```python
from build123d import *

# Parameters (mm, degrees)
SKETCH1_R                        = 5
BOSS_EXTRUDE1_DEPTH              = 34
CHAMFER1_SIZE                    = 0.5
SKETCH2_R                        = 11
BOSS_EXTRUDE2_DEPTH              = 2
SKETCH3_W                        = 3
SKETCH3_H                        = 1.8
CUT_EXTRUDE1_DEPTH               = 12
FILLET1_R                        = 1.5
BOSS_EXTRUDE3_START              = 10
SKETCH4_R                        = 5
BOSS_EXTRUDE3_DEPTH              = 10
SKETCH6_W                        = 0.8
SKETCH6_H                        = 0.5
CHAMFER2_SIZE                    = 0.5
CUT_EXTRUDE2_DEPTH               = 38.389838192
TAP_DRILL_FOR_M4_HELICOIL1_D     = 4.2
TAP_DRILL_FOR_M4_HELICOIL1_DEPTH = 20
TAP_DRILL_FOR_M4_HELICOIL1_TIP   = 1.2618073


with BuildPart() as part:
    # Sketch1 → Boss-Extrude1 (new body)
    with BuildSketch(Plane(origin=(0, 0, 0), x_dir=(0, 0, -1), z_dir=(1, 0, 0))):
        Circle(SKETCH1_R)
    extrude(amount=BOSS_EXTRUDE1_DEPTH)

    # Chamfer1
    chamfer1_edges = [part.edges().sort_by_distance(p)[0] for p in [
        (34, 0, 5),
    ]]
    chamfer(chamfer1_edges, length=CHAMFER1_SIZE)

    # Sketch2 → Boss-Extrude2 (add)
    with BuildSketch(Plane.ZY):
        Circle(SKETCH2_R)
    extrude(amount=BOSS_EXTRUDE2_DEPTH)

    # Sketch3 → Cut-Extrude1 (cut)
    with BuildSketch(Plane(origin=(34, 0, 0), x_dir=(0, 0, -1), z_dir=(1, 0, 0))):
        with Locations((0, 4.1)):
            Rectangle(SKETCH3_W, SKETCH3_H)
    extrude(amount=-CUT_EXTRUDE1_DEPTH, mode=Mode.SUBTRACT)

    # Fillet1
    fillet1_edges = [part.edges().sort_by_distance(p)[0] for p in [
        (22, 3.984848004, 1.5),
        (22, 3.984848004, -1.5),
    ]]
    fillet(fillet1_edges, radius=FILLET1_R - 0.0001)  # a hair under: the kernel refuses the full size

    # Sketch4 → Boss-Extrude3 (add)
    with BuildSketch(Plane.ZY.offset(2).offset(BOSS_EXTRUDE3_START)):
        with Locations(Location((0, 0, 0), (0, 0, 72.542396876))):
            Circle(SKETCH4_R)
    extrude(amount=-BOSS_EXTRUDE3_DEPTH)

    # Sketch6 → Cut-Revolve1 (revolve, cut)
    with BuildSketch(Plane.XY, mode=Mode.PRIVATE) as cut_revolve1_sk:
        with Locations((-2.4, 4.75)):
            Rectangle(SKETCH6_W, SKETCH6_H)
        with Locations((0.4, 4.75)):
            Rectangle(SKETCH6_W, SKETCH6_H)
    revolve(cut_revolve1_sk.sketch.rotate(Axis((0, 0, 0), (1, 0, 0)), 90), axis=Axis((0, 0, 0), (1, 0, 0)), mode=Mode.SUBTRACT)

    # Chamfer2
    chamfer2_edges = [part.edges().sort_by_distance(p)[0] for p in [
        (-12, -4.769696007, -1.5),
    ]]
    chamfer(chamfer2_edges, length=CHAMFER2_SIZE)

    # Sketch7 → Cut-Extrude2 (cut, through all)
    with BuildSketch(Plane(origin=(0, 0, 0), x_dir=(0, 0, -1), z_dir=(1, 0, 0))):
        with BuildLine():
            Line((-4, 3), (-4, -3))
            ThreePointArc((-4, -3), (-5, 0), (-4, 3))
        make_face()
        with BuildLine():
            Line((4, 3), (4, -3))
            ThreePointArc((4, -3), (5, 0), (4, 3))
        make_face()
    extrude(amount=CUT_EXTRUDE2_DEPTH, mode=Mode.SUBTRACT)

    # Tap Drill for M4 Helicoil1
    with Locations(Plane(origin=(34, 0, 0), x_dir=(0, 0, -1), z_dir=(1, 0, 0))):
        with Locations((0, 0)):
            Hole(TAP_DRILL_FOR_M4_HELICOIL1_D / 2, depth=TAP_DRILL_FOR_M4_HELICOIL1_DEPTH)
            with Locations((0, 0, -(TAP_DRILL_FOR_M4_HELICOIL1_DEPTH + TAP_DRILL_FOR_M4_HELICOIL1_TIP / 2))):  # 118° drill point
                Cone(0, TAP_DRILL_FOR_M4_HELICOIL1_D / 2, TAP_DRILL_FOR_M4_HELICOIL1_TIP, mode=Mode.SUBTRACT)


solid = part.part
```
Geometry check sheet. Reference: the model listing, model coordinates, mm. A direction names the side the tool comes from. Give positions to 0.01 mm unless a question says otherwise; leave off trailing zeros. Loops run counter-clockwise (first coordinate to the right, second up) from the corner with the lowest first, then second, coordinate; pieces in that order, holes last. Notation, with made-up numbers: (34, 19.5) - (46, 19.5) arc R21 ccw to (46, 42.5) - close; hole circle Ø7 at (64, -5). An arc over 180 degrees is marked (long way). Use CSV: the item, a comma, the result in double quotes. Start each with the question number.
Q1. Section check C-C, the plane x = 4. Record the cut outline in (y, z), and give its area (3 significant figures).
Q2. Section check B-B, the plane y = 5.5. Record the cut outline in (x, z), and give its area (3 significant figures).
Q3. Section check A-A, the plane x = 25. Record the cut outline in (y, z), and give its area (3 significant figures).
Q4. Scan lines: probe 1 along Z at (x, y) = (19.75, 0); probe 2 along Z at (x, y) = (24, 4); probe 3 along X at (y, z) = (8, 5.75). Record each from-to range of solid material in increasing order. Write a range as from..to.
Q5. Access from +Z, -Z, +X, -X, +Y, -Y to the whole of each face (thin tool, end or side, straight path). Record for faces 4 (the face through (-2.39, -3.04, -3.32)), 5 (the face through (0.4, -4.5, 0.1)), 6 (the face through (0.4, 4.5, -0.1)), 7 (the face through (23.86, 0.631, 2.003)).
Q6. Go/stop test with flat-tipped pins: pin 1 Ø2 at (x, y) = (1.5, 3) entering from -Z; pin 2 Ø5 at (x, y) = (26, -0.5) entering from +Z; pin 3 Ø2 at (x, z) = (24, 0.5) entering from -Y. Record where each tip stops, or that it passes through.
Q7. Release check for a two-part mould opening along X. For faces 1 (the face through (-12, 0, 0)), 2 (the face through (0.8, 4.7, 0)), 3 (the face through (29, 4, -1.5)) record: +X half, -X half, draft (parallel to the pull), parting line (faces both ways), or undercut.
Findings below:
1,outline,"(-3, -4) - (3, -4) arc R5 ccw to (3, 4) - (-3, 4) arc R5 ccw to start"
1,area,"70.4 mm^2"
2,outline,"(-2, -9.53) - (0, -9.53) - (0, 9.53) - (-2, 9.53) - close"
2,area,"38.1 mm^2"
3,outline,"(-3, -4) - (3, -4) arc R5 ccw to (4.77, -1.5) - (3.2, -1.5) - (3.2, 1.5) - (4.77, 1.5) arc R5 ccw to (3, 4) - (-3, 4) arc R5 ccw to start; hole circle Ø4.2 at (0, 0)"
3,area,"51.3 mm^2"
4,probe 1,"z = -4..-2.1, 2.1..4"
4,probe 2,"z = -3..-1.5, 1.5..3"
4,probe 3,"x = -2..0"
5,face 4,"none"
5,face 5,"-Y"
5,face 6,"+Y"
5,face 7,"+X"
6,pin 1,"stops at z = -4"
6,pin 2,"stops at z = 4"
6,pin 3,"stops at y = -5"
7,face 1,"-X half"
7,face 2,"undercut"
7,face 3,"draft"
